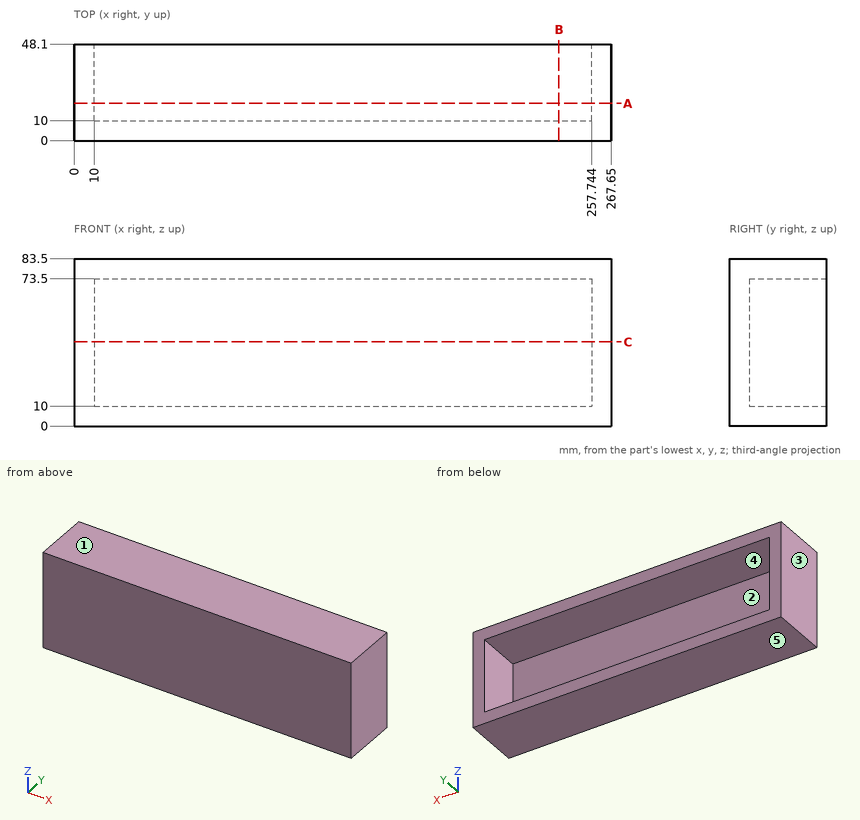
Job drawing, mm, ordinate dimensions from the low corner. One solid piece. A direction names the side the tool comes from. Coordinates: 2 decimals unless noted, no trailing zeros. Write each loop counter-clockwise with the first axis right and the second up, starting at its lowest first coordinate (ties: lowest second). Pieces come first, ordered by that corner, then holes. Notation, with made-up numbers: M 49.5,-10.75 L 102.5,-10.75 A7 ccw 102.5,-2.75 Z; hole C 18.5,-31.5 d1. An arc over 180 degrees is marked long. Answer as a JSON object with one key per item and string values. Group by question number.
1) Wall check: line 1 (X direction, y = 34.5, z = 12); line 2 (Z direction, x = 249.5, y = 25); line 3 (Y direction, x = 58.5, z = 20). Give the ranges that are in metal, low to high. Write a range as from..to.
2) Saw through at B-B (x = 241.5). Write the cut outline in (y, z), plus the area to 3 significant figures.
3) Saw through at C-C (z = 42). Write the cut outline in (x, y).
4) Tool access for the marked faces 1 and 2: list every direction of +Z, -Z, +X, -X, +Y, -Y with a clear straight run to the whole face (end or side of a thin tool).
5) Saw through at A-A (y = 18.5). Write the cut outline in (x, z).
6) Pin check, flat tip, straight feed: pin 1 Ø19 at (x, z) = (118.5, 53.5) entering from +Y. Stop position of the tip, or through.
7) Mould opens along Z. For the marked faces 3, 4 and 5 say: +Z half, -Z half, draft (parallel to the pull), parting line (faces both ways), or undercut.
Values follow:
{
 "1": {"line 1": "x = 0..10, 257.74..267.65", "line 2": "z = 0..10, 73.5..83.5", "line 3": "y = 0..10"},
 "2": {"outline": "M 0,0 L 48.1,0 L 48.1,10 L 10,10 L 10,73.5 L 48.1,73.5 L 48.1,83.5 L 0,83.5 Z", "area": "1,600 mm2"},
 "3": {"outline": "M 0,0 L 267.65,0 L 267.65,48.1 L 257.74,48.1 L 257.74,10 L 10,10 L 10,48.1 L 0,48.1 Z"},
 "4": {"face 1": "+Z, +X, -X, +Y, -Y", "face 2": "+Y"},
 "5": {"outline": "M 0,0 L 267.65,0 L 267.65,83.5 L 0,83.5 Z; hole M 10,10 L 257.74,10 L 257.74,73.5 L 10,73.5 Z"},
 "6": {"pin 1": "stops at y = 10"},
 "7": {"face 3": "draft", "face 4": "undercut", "face 5": "-Z half"}
}
